Work out the finished part from the listing and answer in its coordinate system (mm). Face numbers are marked on the shaded views. A direction names the side the tool comes from. Give positions to 0.01 mm unless a question says otherwise; leave off trailing zeros. Loops run counter-clockwise (first coordinate to the right, second up) from the corner with the lowest first, then second, coordinate; pieces in that order, holes last. Notation, with made-up numbers: M 52.25,15 L 77.25,15 A25 cw 77.25,41 Z; hole C -23.5,26 d6. An arc over 180 degrees is marked long. Use a Markdown table: item, result.
```python
from build123d import *

# Parameters (mm, degrees)
SKETCH1_R           = 1.7
SKETCH1_R_2         = 1.0922
BOSS_EXTRUDE1_DEPTH = 6.35


with BuildPart() as part:
    # Sketch1 → Boss-Extrude1 (new body)
    with BuildSketch(Plane(origin=(0, 0, 0), x_dir=(1, 0, 0), z_dir=(0, 1, 0))):
        Polygon((32.881906518, 19.245524772), (-0.226160103, 38.099328755), (-33.108066621, 18.853803983), (-32.881906518, -19.245524772), (0.226160103, -38.099328755), (33.108066621, -18.853803983), align=None)
        with Locations(Location((-13.553347751, 22.99968689, 0), (0, 0, 270))):
            Circle(SKETCH1_R, mode=Mode.SUBTRACT)
        with Locations(Location((13.14163925, 23.237386904, 0), (0, 0, 270))):
            Circle(SKETCH1_R, mode=Mode.SUBTRACT)
        with Locations(Location((26.694987002, 0.237700014, 0), (0, 0, 270))):
            Circle(SKETCH1_R, mode=Mode.SUBTRACT)
        with Locations(Location((13.553347751, -22.99968689, 0), (0, 0, 270))):
            Circle(SKETCH1_R, mode=Mode.SUBTRACT)
        with Locations(Location((-13.14163925, -23.237386904, 0), (0, 0, 270))):
            Circle(SKETCH1_R, mode=Mode.SUBTRACT)
        with Locations(Location((-26.694987002, -0.237700014, 0), (0, 0, 270))):
            Circle(SKETCH1_R, mode=Mode.SUBTRACT)
        with Locations(Location((-30.248450738, 17.202803983, 0), (0, 0, 270))):
            Circle(SKETCH1_R_2, mode=Mode.SUBTRACT)
        with Locations(Location((-0.226160103, 34.797328755, 0), (0, 0, 270))):
            Circle(SKETCH1_R_2, mode=Mode.SUBTRACT)
        with Locations(Location((30.022290634, 17.594524772, 0), (0, 0, 270))):
            Circle(SKETCH1_R_2, mode=Mode.SUBTRACT)
        with Locations(Location((30.248450738, -17.202803983, 0), (0, 0, 270))):
            Circle(SKETCH1_R_2, mode=Mode.SUBTRACT)
        with Locations(Location((0.226160103, -34.797328755, 0), (0, 0, 270))):
            Circle(SKETCH1_R_2, mode=Mode.SUBTRACT)
        with Locations(Location((-30.022290634, -17.594524772, 0), (0, 0, 270))):
            Circle(SKETCH1_R_2, mode=Mode.SUBTRACT)
        Polygon((3.825955971, 24.566392182), (7.031797703, 22.753364938), (10.345261287, 28.61231707), (7.139419555, 30.425344314), align=None, mode=Mode.SUBTRACT)
        Polygon((-10.853125511, 28.4235604), (-7.435855918, 22.624540696), (-4.262807401, 24.494367455), (-7.680076994, 30.293387159), align=None, mode=Mode.SUBTRACT)
        Polygon((15.875499033, 17.751910472), (19.081340765, 15.938883228), (22.394804349, 21.797835359), (19.188962617, 23.610862603), align=None, mode=Mode.SUBTRACT)
        Polygon((23.188097695, 8.969821027), (23.22089091, 5.286967024), (29.951624087, 5.346899452), (29.918830872, 9.029753454), align=None, mode=Mode.SUBTRACT)
        Polygon((-19.362141724, 15.596571155), (-16.189093207, 17.466397914), (-19.6063628, 23.265417618), (-22.779411317, 21.395590859), align=None, mode=Mode.SUBTRACT)
        Polygon((23.311354951, -4.872630224), (23.344148166, -8.555484227), (30.074881343, -8.4955518), (30.042088128, -4.812697797), align=None, mode=Mode.SUBTRACT)
        Polygon((19.362141724, -15.596571155), (16.189093207, -17.466397914), (19.6063628, -23.265417618), (22.779411317, -21.395590859), align=None, mode=Mode.SUBTRACT)
        Polygon((7.435855918, -22.624540696), (4.262807401, -24.494367455), (7.680076994, -30.293387159), (10.853125511, -28.4235604), align=None, mode=Mode.SUBTRACT)
        Polygon((-3.825955971, -24.566392182), (-7.031797703, -22.753364938), (-10.345261287, -28.61231707), (-7.139419555, -30.425344314), align=None, mode=Mode.SUBTRACT)
        Polygon((-15.875499033, -17.751910472), (-19.081340765, -15.938883228), (-22.394804349, -21.797835359), (-19.188962617, -23.610862603), align=None, mode=Mode.SUBTRACT)
        Polygon((-23.188097695, -8.969821027), (-23.22089091, -5.286967024), (-29.951624087, -5.346899452), (-29.918830872, -9.029753454), align=None, mode=Mode.SUBTRACT)
        Polygon((-23.311354951, 4.872630224), (-23.344148166, 8.555484227), (-30.074881343, 8.4955518), (-30.042088128, 4.812697797), align=None, mode=Mode.SUBTRACT)
        Polygon((-13.367735769, 20.308263579), (-11.288841912, 21.53332249), (-8.129479458, 16.17196465), (-10.208373314, 14.946905739), align=None, mode=Mode.SUBTRACT)
        Polygon((10.903604282, 21.730930556), (13.003983348, 20.54308512), (9.940592487, 15.126318055), (7.840213421, 16.314163491), align=None, mode=Mode.SUBTRACT)
        Polygon((24.27134005, 1.422666977), (24.29282526, -0.990237369), (18.070071945, -1.045646595), (18.048586735, 1.367257752), align=None, mode=Mode.SUBTRACT)
        Polygon((13.367735769, -20.308263579), (11.288841912, -21.53332249), (8.129479458, -16.17196465), (10.208373314, -14.946905739), align=None, mode=Mode.SUBTRACT)
        Polygon((-10.903604282, -21.730930556), (-13.003983348, -20.54308512), (-9.940592487, -15.126318055), (-7.840213421, -16.314163491), align=None, mode=Mode.SUBTRACT)
        Polygon((-24.27134005, -1.422666977), (-24.29282526, 0.990237369), (-18.070071945, 1.045646595), (-18.048586735, -1.367257752), align=None, mode=Mode.SUBTRACT)
        Polygon((15.732581095, 9.344357123), (-0.226160103, 18.296993457), (-15.958741198, 8.952636334), (-15.732581095, -9.344357123), (0.226160103, -18.296993457), (15.958741198, -8.952636334), align=None, mode=Mode.SUBTRACT)
    extrude(amount=-BOSS_EXTRUDE1_DEPTH)


solid = part.part
```
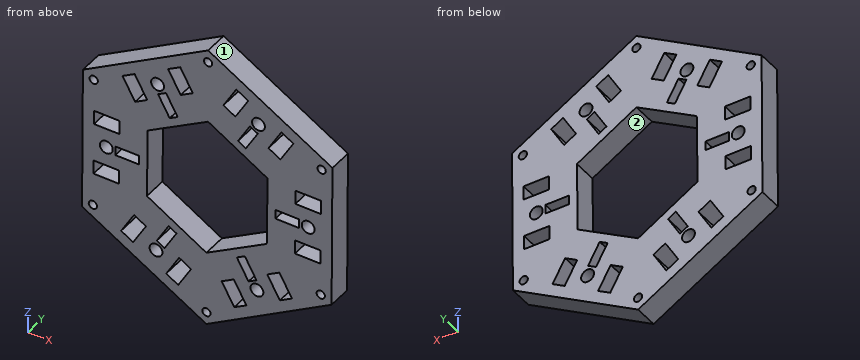
(1) Which of the six approach directions +Z, -Z, +X, -X, +Y, -Y give full straight-line access (tool end or side, diameter ignored) to the marked faces 1 and 2?
Entries:
| item | result |
|---|---|
| face 1 | +Z, +X, +Y, -Y |
| face 2 | +Y, -Y |
(2) A cutting plane is placed at C-C (y = -1). Count the separate pieces of the cut face and the enclosed holes in it, and give its area (3 significant figures).
Entries:
| item | result |
|---|---|
| separate pieces | 1 |
| enclosed holes | 31 |
| area | 2,440 mm² |
(3) A cutting plane is placed at A-A (z = 3). Write down the section's boundary in (x, y), and give its area (3 significant figures).
Entries:
| item | result |
|---|---|
| outline | M -32.98,-6.35 L -15.81,-6.35 L -15.81,0 L -32.98,0 Z; M 15.89,-6.35 L 33.01,-6.35 L 33.01,0 L 15.89,0 Z |
| area | 218 mm² |
(4) Consider probe 1 along Z at (x, y) = (25.5, -0.75); probe 2 along Z at (x, y) = (17, -2); probe 3 along X at (y, z) = (-4, 7). Determine where each line is inside the solid, lowest interval first. Write a range as [from, to].
Entries:
| item | result |
|---|---|
| probe 1 | z = [-23.45, -8.99], [-5.31, -1.45], [0.97, 4.85], [8.54, 23.31] |
| probe 2 | z = [-28.29, -19.74], [-17.12, 16.99], [18.84, 28.28] |
| probe 3 | x = [-32.95, -29.94], [-23.21, -15.76], [15.93, 23.33], [30.06, 33.04] |
(5) A cutting plane is placed at B-B (x = -5.5). Write down the section's boundary in (y, z), and give its area (3 significant figures).
Entries:
| item | result |
|---|---|
| outline | M -6.35,-35.01 L 0,-35.01 L 0,-26.59 L -6.35,-26.59 Z; M -6.35,-23.77 L 0,-23.77 L 0,-15.16 L -6.35,-15.16 Z; M -6.35,15.08 L 0,15.08 L 0,23.62 L -6.35,23.62 Z; M -6.35,27.53 L 0,27.53 L 0,34.84 L -6.35,34.84 Z |
| area | 209 mm² |
(6) Given P1, Ø1, axis at x = 16, z = -8.5, coming from the +Y side; P2, Ø1.3, axis at x = 30.25, z = 17.2, coming from the +Y side; P3, Ø1.5, axis at y = -3.5, z = 27, coming from the -X side; P4, Ø1, axis at y = -4.5, z = -27, coming from the +X side, each flat-ended and moving along its own axis, determine where each tip first touches the part or whether it passes through.
Entries:
| item | result |
|---|---|
| P1 | stops at y = 0 |
| P2 | passes through |
| P3 | stops at x = -20.58 |
| P4 | stops at x = 20.14 |
